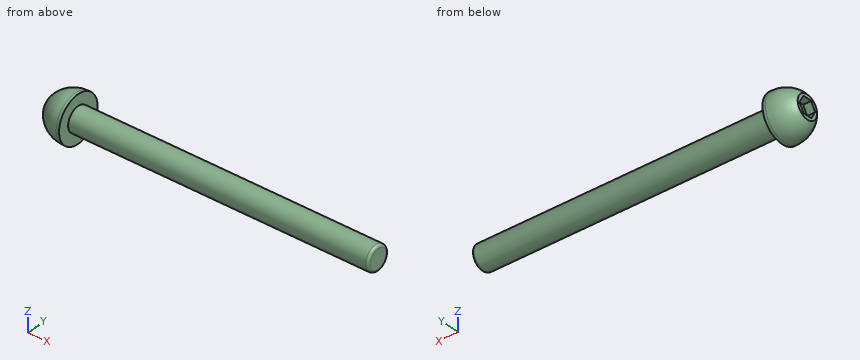
```python
from build123d import *

# Parameters (mm, degrees)
CONG_1_R                = 0.3
ENL_V_MAT_EXTRU_1_DEPTH = 1


with BuildPart() as part:
    # Esquisse1 → Révolution1 (revolve)
    with BuildSketch(Plane.XY):
        with BuildLine():
            Line((40.164888985, 0), (0, 0))
            Line((0, 0), (0, 1.43))
            ThreePointArc((0, 1.43), (1.238500708, 2.474899998), (2.814888985, 2.85))
            Line((2.814888985, 2.85), (3.164888985, 2.85))
            Line((3.164888985, 2.85), (3.164888985, 1.5))
            Line((3.164888985, 1.5), (40.164888985, 1.5))
            Line((40.164888985, 1.5), (40.164888985, 0))
        make_face()
    revolve(axis=Axis((40.164888985, 0, 0), (-1, 0, 0)))

    # Congé1
    cong_1_edges = [part.edges().sort_by_distance(p)[0] for p in [
        (40.164888985, -1.5, 0),
    ]]
    fillet(cong_1_edges, radius=CONG_1_R)

    # Esquisse2 → Enlèv. mat.-Extru.1 (cut)
    with BuildSketch(Plane.ZY):
        Polygon((0, 1.154700538), (-1, 0.577350269), (-1, -0.577350269), (0, -1.154700538), (1, -0.577350269), (1, 0.577350269), align=None)
    extrude(amount=-ENL_V_MAT_EXTRU_1_DEPTH, mode=Mode.SUBTRACT)


solid = part.part
```
Verification items for the finished model (mm, model axes). Coordinates: 2 decimals unless noted, no trailing zeros. Write each loop counter-clockwise with the first axis right and the second up, starting at its lowest first coordinate (ties: lowest second). Pieces come first, ordered by that corner, then holes. Notation, with made-up numbers: M -6.5,-15.75 L 15.5,-15.75 A37 ccw 15.5,21.25 Z; hole C 77,-19.5 d5. An arc over 180 degrees is marked long. Answer as a JSON object with one key per item and string values. Group by question number.
(1) Gauge pin test, flat ends, axial feed: pin 1 (1.1 mm diameter, centred on x = 0.5, y = 0, fed in from +Z); pin 2 (1.1 mm diameter, centred on x = 0.5, y = 0, fed in from -Z); pin 3 (2 mm diameter, centred on x = 23.5, y = 0.5, fed in from -Z). Record the tip position at first contact, or that the pin passes through.
(2) Cross-section at A-A, the plane x = 32.5. Record the cut outline in (y, z).
(3) Material ranges on line 1 (Z direction, x = 20.5, y = -0.15); line 2 (X direction, y = -0.4, z = -0.65); line 3 (Y direction, x = 22.5, z = 0.6), recorded low to high.
Reply:
{
 "1": {"pin 1": "z = 2.37", "pin 2": "z = -2.37", "pin 3": "z = -1.5"},
 "2": {"outline": "C 0,0 d3"},
 "3": {"line 1": "-1.49 to 1.49", "line 2": "1 to 40.16", "line 3": "-1.37 to 1.37"}
}
